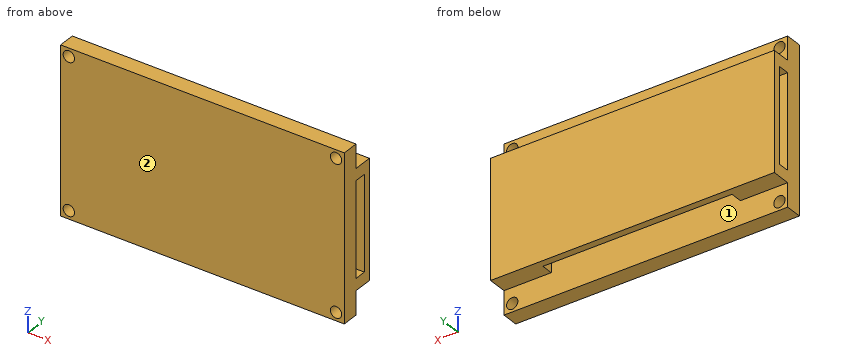
```python
from build123d import *

# Parameters (mm, degrees)
CROQUIS1_W                   = 120
CROQUIS1_H                   = 70
SALIENTE_EXTRUIR1_DEPTH      = 7
TALADRO_DE_MARGEN_PARA_M41_D = 4.8
CROQUIS8_W                   = 120
CROQUIS8_H                   = 5
SALIENTE_EXTRUIR2_DEPTH      = 5
CROQUIS9_W                   = 120
CROQUIS9_H                   = 50
SALIENTE_EXTRUIR3_DEPTH      = 3
CROQUIS10_W                  = 80
CROQUIS10_H                  = 5
CORTAR_EXTRUIR1_DEPTH        = 87.168439698


with BuildPart() as part:
    # Croquis1 → Saliente-Extruir1 (new body)
    with BuildSketch(Plane(origin=(0, 0, 0), x_dir=(1, 0, 0), z_dir=(0, 1, 0))):
        Rectangle(CROQUIS1_W, CROQUIS1_H)
    extrude(amount=SALIENTE_EXTRUIR1_DEPTH)

    # Taladro de margen para M41 (through all)
    with Locations(Plane(origin=(0, 7, 0), x_dir=(1, 0, 0), z_dir=(0, 1, 0))):
        with Locations((56.5, 31.5), (56.5, -31.5), (-56.5, -31.5), (-56.5, 31.5)):
            Hole(TALADRO_DE_MARGEN_PARA_M41_D / 2)

    # Croquis8 → Saliente-Extruir2 (add)
    with BuildSketch(Plane(origin=(0, 7, 0), x_dir=(1, 0, 0), z_dir=(0, 1, 0))):
        with Locations((0, 22.5)):
            Rectangle(CROQUIS8_W, CROQUIS8_H)
        with Locations((0, -22.5)):
            Rectangle(CROQUIS8_W, CROQUIS8_H)
    extrude(amount=SALIENTE_EXTRUIR2_DEPTH)

    # Croquis9 → Saliente-Extruir3 (add)
    with BuildSketch(Plane(origin=(0, 12, 0), x_dir=(1, 0, 0), z_dir=(0, 1, 0))):
        Rectangle(CROQUIS9_W, CROQUIS9_H)
    extrude(amount=SALIENTE_EXTRUIR3_DEPTH)

    # Croquis10 → Cortar-Extruir1 (cut, through all)
    with BuildSketch(Plane.XY.offset(25)):
        with Locations((0, 9.5)):
            Rectangle(CROQUIS10_W, CROQUIS10_H)
    extrude(amount=-CORTAR_EXTRUIR1_DEPTH, mode=Mode.SUBTRACT)


solid = part.part
```
Work out the finished part from the listing and answer in its coordinate system (mm). Face numbers are marked on the shaded views. Coordinates: 2 decimals unless noted, no trailing zeros. Loops run counter-clockwise (first coordinate to the right, second up) from the corner with the lowest first, then second, coordinate; pieces in that order, holes last.
1) Section B-B (x = 56.5) is taken. Give the vertices of the cut face in (y, z), plus the area to 3 significant figures.
Results:
outline: (0, -35) - (7, -35) - (7, -33.9) - (0, -33.9) - close; (0, -29.1) - (7, -29.1) - (7, -25) - (15, -25) - (15, 25) - (7, 25) - (7, 29.1) - (0, 29.1) - close; (0, 33.9) - (7, 33.9) - (7, 35) - (0, 35) - close; hole (7, -20) - (12, -20) - (12, 20) - (7, 20) - close
area: 623 mm2
2) Section D-D (z = 31.5) is taken. Give the vertices of the cut face in (x, y), plus the area to 3 significant figures.
Results:
outline: (-60, 0) - (-58.9, 0) - (-58.9, 7) - (-60, 7) - close; (-54.1, 0) - (54.1, 0) - (54.1, 7) - (-54.1, 7) - close; (58.9, 0) - (60, 0) - (60, 7) - (58.9, 7) - close
area: 773 mm2
3) Section A-A (z = -2.5) is taken. Give the vertices of the cut face in (x, y).
Results:
outline: (-60, 0) - (60, 0) - (60, 7) - (-60, 7) - close; (-60, 12) - (60, 12) - (60, 15) - (-60, 15) - close
4) For a pull along Z with two mould halves and no side action, classify the marked faces 1 and 2 as +Z half, -Z half, draft (parallel to the pull), parting line (faces both ways), or undercut.
Results:
face 1: undercut
face 2: draft
5) Section C-C (x = -31.5) is taken. Give the vertices of the cut face in (y, z).
Results:
outline: (0, -35) - (7, -35) - (7, 35) - (0, 35) - close; (12, -25) - (15, -25) - (15, 25) - (12, 25) - close
6) Flat-ended cylindrical pins translate along their axes: pin 1 (2.5 mm diameter, centred on x = 20.5, y = 12, fed in from -Z); pin 2 (1.5 mm diameter, centred on x = 51.5, y = 10.5, fed in from +Z); pin 3 (3 mm diameter, centred on x = -56.5, z = 31.5, fed in from -Y). Find the tip coordinate at first contact, or state that the pin passes through.
Results:
pin 1: stops at z = -25
pin 2: stops at z = 25
pin 3: passes through
7) Consider probe 1 along X at (y, z) = (5, 31.5); probe 2 along Z at (x, y) = (-56.5, 2.5); probe 3 along Y at (x, z) = (28, -10). Determine where each line is inside the solid, lowest interval first.
Results:
probe 1: x = -60 to -58.9, -54.1 to 54.1, 58.9 to 60
probe 2: z = -35 to -33.9, -29.1 to 29.1, 33.9 to 35
probe 3: y = 0 to 7, 12 to 15
